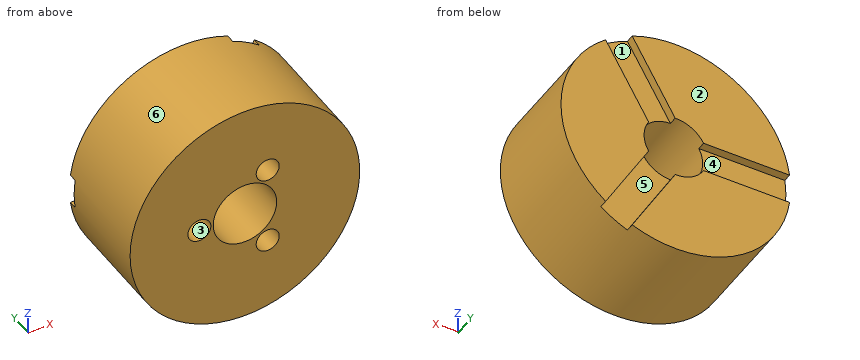
Autodesk Inventor part; units mm, degrees
ref_plane "XZ Plane" through (0, 0, 0) normal (0, 1, 0) x (-1, 0, 0)
sketch "Sketch1" plane through (0, 0, 0) normal (0, 1, 0) x (-1, 0, 0)
  circle A0 centre (0, 0) radius 99.7
extrude "Extrusion1" add sketch "Sketch1" along normal blind 90.9
sketch "Sketch2" plane through (0, 90.9, 0) normal (0, 1, 0) x (1, 0, 0)
  circle A0 centre (0, 0) radius 27.56
  dimension "d3" = 55.12
extrude "Extrusion2" cut sketch "Sketch2" against normal blind 90.9
sketch "Sketch3" plane through (0, 90.9, 0) normal (0, 1, 0) x (1, 0, 0)
  circle A0 centre (0, 0) radius 99.7
  line L0 (-99.7, 0) -> (-98.8062, 13.32)
  line L1 (-98.8062, 13.32) -> (-24.1274, 13.32)
  circle A1 centre (0, 0) radius 27.56
  line L2 (-99.7, 0) -> (-98.8062, -13.32)
  line L3 (-98.8062, -13.32) -> (-24.1274, -13.32)
  line L4 (37.8676, -92.2287) -> (0.5282, -27.5549)
  line L5 (49.85, -86.3427) -> (37.8676, -92.2287)
  line L6 (49.85, -86.3427) -> (60.9386, -78.9087)
  line L7 (60.9386, -78.9087) -> (23.5992, -14.2349)
  line L8 (60.9386, 78.9087) -> (23.5992, 14.2349)
  line L9 (49.85, 86.3427) -> (60.9386, 78.9087)
  line L10 (49.85, 86.3427) -> (37.8676, 92.2287)
  line L11 (37.8676, 92.2287) -> (0.5282, 27.5549)
  line L12 (-24.1274, 13.32) -> (-24.1274, -13.32)
  line L13 (0.5282, 27.5549) -> (23.5992, 14.2349)
  line L14 (23.5992, -14.2349) -> (0.5282, -27.5549)
  dimension "d6" = 13.35
  dimension "d15" = 360
ref_plane "Work Plane2" through (-99.7, 83.72, 0) normal (0.9978, 0, 0.067) x (0.067, 0, -0.9978)
sketch "Sketch4" plane through (-99.7, 83.72, 0) normal (0.9978, 0, 0.067) x (0.067, 0, -0.9978)
  line L0 (13.35, 0) -> (13.35, 7.18)
  line L1 (-13.2303, 7.18) -> (-13.2303, 0)
  point P0 (6.675, -83.72)
ref_plane "Work Plane1" through (-98.8062, 83.72, 13.32) normal (0.9978, 0, -0.067) x (-0.067, 0, -0.9978)
sketch "Sketch5" plane through (-98.8062, 83.72, 13.32) normal (0.9978, 0, -0.067) x (-0.067, 0, -0.9978)
  line L0 (13.35, 0) -> (13.35, 7.18)
  line L1 (0, 0) -> (13.35, 0)
  line L2 (13.35, 5.7337) -> (13.35, 0)
  line L3 (13.35, 0) -> (0, 0)
  line L4 (0, 0) -> (0, 7.18)
  line L5 (0, 7.18) -> (0, 0)
  line L6 (106.375, 7.18) -> (-93.025, 7.18)
  point P0 (6.675, -83.72)
  point P1 (26.5803, 7.18)
extrude "Extrusion4" cut sketch "Sketch5" against normal blind 7.18
ref_plane "Work Plane3" through (-99.7, 83.72, 0) normal (0.9978, 0, 0.067) x (0.067, 0, -0.9978)
sketch "Sketch6" plane through (-99.7, 83.72, 0) normal (0.9978, 0, 0.067) x (0.067, 0, -0.9978)
  line L0 (0, 0) -> (13.35, 0)
  line L1 (0, 0) -> (0, 7.18)
  line L2 (0, 0) -> (0, 7.18)
  line L3 (13.35, 7.18) -> (18.3498, 7.18)
  line L4 (0, 7.18) -> (13.35, 7.18)
  line L5 (13.35, 0) -> (13.35, 7.18)
  line L6 (13.35, 7.18) -> (13.35, 0)
  line L7 (13.35, 0) -> (0, 0)
  point P0 (6.675, -83.72)
extrude "Extrusion5" cut sketch "Sketch6" against normal blind 7.18
extrude "Extrusion6" cut sketch "Sketch3" against normal blind 7.18 contours L8 A1 L11 L10 L9 | L6 L5 L4 A1 L7 | L13 A1 | A1 L14 | L1 A1 L3 L2 L0
sketch "Sketch7" plane through (49.85, 83.72, -86.3427) normal (-0.5569, 0, 0.8306) x (0.8306, 0, 0.5569)
  line L0 (13.35, 7.18) -> (0, 7.18)
  line L1 (13.35, 0) -> (13.35, 7.18)
  line L2 (0, 7.18) -> (13.35, 7.18)
  line L3 (13.35, 0) -> (18.3498, 0)
  line L4 (13.35, 7.18) -> (13.35, 0)
  line L5 (0, 7.18) -> (0, 0)
  line L6 (13.35, 0) -> (0, 0)
  line L7 (0, 0) -> (0, 6.2119)
  line L8 (0, 7.18) -> (-13.2303, 7.18)
  line L9 (-13.2303, 4.6736) -> (0, 7.18)
  line L10 (0, 7.18) -> (0, 0)
  line L11 (-13.2303, -2.9965) -> (-13.2303, 4.6736)
  line L12 (-13.2303, 0) -> (-13.2303, 7.18)
  point P0 (6.675, -83.72)
extrude "Extrusion7" cut sketch "Sketch7" against normal blind 10 contours L1 L6 L5 L0
sketch "Sketch8" plane through (37.8676, 83.72, -92.2287) normal (-0.4409, 0, 0.8976) x (0.8976, 0, 0.4409)
  line L0 (0, 0) -> (0, 7.18)
  line L1 (-4.9998, 0) -> (0, 0)
  line L2 (0, 7.18) -> (0, 0)
  line L3 (0, 0) -> (13.35, 0)
  line L4 (0, 0) -> (13.35, 0)
  line L5 (13.35, 7.18) -> (13.35, 0)
  line L6 (13.35, 0) -> (13.35, 7.18)
  line L7 (0, 7.18) -> (13.35, 7.18)
  line L8 (13.35, 7.18) -> (0, 7.18)
  line L9 (0, 7.18) -> (0, 4.7035)
  point P0 (6.675, -83.72)
extrude "Extrusion8" cut sketch "Sketch8" against normal blind 10
sketch "Sketch10" plane through (49.85, 83.72, 86.3427) normal (-0.4409, 0, -0.8976) x (-0.8976, 0, 0.4409)
  line L0 (0, 7.18) -> (13.35, 7.18)
  line L1 (13.35, 7.18) -> (18.3498, 7.18)
  line L2 (0, 7.18) -> (13.35, 7.18)
  line L3 (13.35, 0) -> (18.3498, 0)
  line L4 (13.35, 7.18) -> (13.35, 0)
  line L5 (0, 0) -> (13.35, 0)
  line L6 (13.35, 0) -> (0, 0)
  line L7 (0, 0) -> (0, 7.18)
  line L8 (0, 7.18) -> (0, 0)
  point P0 (6.675, -83.72)
extrude "Extrusion9" cut sketch "Sketch10" against normal blind 10
sketch "Sketch11" plane through (60.9386, 83.72, 78.9087) normal (-0.5569, 0, -0.8306) x (-0.8306, 0, 0.5569)
  line L0 (-4.9998, 7.18) -> (0, 7.18)
  line L1 (13.35, 7.18) -> (0, 7.18)
  line L2 (0, 7.18) -> (13.35, 7.18)
  line L3 (0, 0) -> (13.35, 0)
  line L4 (13.35, 7.18) -> (13.35, 0)
  line L5 (13.35, 0) -> (0, 0)
  line L6 (0, 0) -> (0, 7.18)
  line L7 (0, 0) -> (0, 7.18)
  point P0 (6.675, -83.72)
extrude "Extrusion10" cut sketch "Sketch11" against normal blind 10
sketch "Sketch12" plane through (0, 90.9, 0) normal (0, 1, 0) x (1, 0, 0)
  arc A0 (37.8676, -92.2287) -> (60.9386, -78.9087) centre (0, 0) ccw
  arc A1 (-98.8062, -13.32) -> (37.8676, -92.2287) centre (0, 0) ccw
  arc A2 (-98.8062, 13.32) -> (-98.8062, -13.32) centre (0, 0) ccw
  arc A3 (37.8676, 92.2287) -> (-98.8062, 13.32) centre (0, 0) ccw
  arc A4 (60.9386, 78.9087) -> (37.8676, 92.2287) centre (0, 0) ccw
  arc A5 (60.9386, -78.9087) -> (60.9386, 78.9087) centre (0, 0) ccw
  circle A6 centre (0, 0) radius 99.7
ref_plane "Work Plane5" through (-99.7, 0, 0) normal (1, 0, 0) x (0, 1, 0)
ref_plane "Work Plane6" through (0, 0, -99.7) normal (0, 0, 1) x (1, 0, 0)
sketch "Sketch13" plane through (0, 83.72, 0) normal (0, 1, 0) x (1, 0, 0)
  arc A0 (60.9386, 78.9087) -> (37.8676, 92.2287) centre (0, 0) ccw
sketch "Sketch14" plane through (-99.7, 83.72, 0) normal (0.9978, 0, 0.067) x (0.067, 0, -0.9978)
  point P0 (6.675, -83.72)
sketch "Sketch15" plane through (0, 0, 0) normal (0, -1, 0) x (1, 0, 0)
  circle A0 centre (0, 0) radius 27.56
  circle A1 centre (19.78, 34.26) radius 10
  circle A2 centre (-39.56, 0) radius 10
  circle A3 centre (19.78, -34.26) radius 10
  point P0 (0.5282, 27.5549)
  point P1 (23.5992, 14.2349)
  dimension "d32" = 360
extrude "Extrusion11" cut sketch "Sketch15" against normal blind 40 contours A1 | A2 | A3
properties part number "3 jaww"
Model file for the job. Use its own axes, mm. Face numbers are marked on the shaded views. A direction names the side the tool comes from. Give positions to 0.01 mm unless a question says otherwise; leave off trailing zeros. Write each loop counter-clockwise with the first axis right and the second up, starting at its lowest first coordinate (ties: lowest second). Pieces come first, ordered by that corner, then holes. Notation, with made-up numbers: (4.25, 40) - (41.25, 40) arc R34 cw to (41.25, 73) - close; hole circle Ø11 at (15.5, 56.25). An arc over 180 degrees is marked (long way). Answer as CSV lines item,"result".
1. Band-saw the part on A-A (x = 19.78). Write the cut outline in (y, z).
Responses:
outline,"(0, -97.72) - (90.9, -97.72) - (90.9, -60.9) - (83.72, -60.9) - (83.72, -19.19) - (0, -19.19) - (0, -24.26) - (40, -24.26) - (40, -44.26) - (0, -44.26) - close; (0, 19.19) - (83.72, 19.19) - (83.72, 60.9) - (90.9, 60.9) - (90.9, 97.72) - (0, 97.72) - (0, 44.26) - (40, 44.26) - (40, 24.26) - (0, 24.26) - close"
2. Two-plate mould, pull along X, no slides. Class the marked faces 4, 5 and 6: +X half, -X half, draft (parallel to the pull), parting line (faces both ways), or undercut.
Responses:
face 4,"draft"
face 5,"undercut"
face 6,"parting line"
3. Drill centre lines: L1, parallel to Z at x = 19.78, y = 31; L2, parallel to Z at x = 18, y = 19; L3, parallel to X at y = 13, z = 41. Where is each one in solid material? Low to high. Write a range as [from, to].
Responses:
L1,"z = [-97.72, -44.26], [-24.26, -19.19], [19.19, 24.26], [44.26, 97.72]"
L2,"z = [-98.06, -44.1], [-24.42, -20.87], [20.87, 24.42], [44.1, 98.06]"
L3,"x = [-90.88, 12.39], [27.17, 90.88]"
4. Band-saw the part on B-B (y = 18). Write the cut outline in (x, z).
Responses:
outline,"circle Ø199.4 at (0, 0); hole circle Ø20 at (-39.56, 0); hole circle Ø55.12 at (0, 0); hole circle Ø20 at (19.78, -34.26); hole circle Ø20 at (19.78, 34.26)"
5. Band-saw the part on D-D (y = 48). Write the cut outline in (x, z), and give its area (3 significant figures).
Responses:
outline,"circle Ø199.4 at (0, 0); hole circle Ø55.12 at (0, 0)"
area,"28,800 mm2"
6. 3-axis set-ups, long thin cutter, end or side, ignore diameter. For the marked faces 1, 2 and 3: which of +Z, -Z, +X, -X, +Y, -Y reach the whole face in a straight line?
Responses:
face 1,"+Y"
face 2,"+Z, -Z, +X, -X, +Y"
face 3,"-Y"
7. Pin check, flat tips, straight feed: pin 1 (6 mm diameter, centred on x = 19, z = -30.5, fed in from -Y); pin 2 (23 mm diameter, centred on x = -39.56, z = 0, fed in from +Y); pin 3 (2 mm diameter, centred on x = -75.5, y = 87.5, fed in from +Z). Stop position of each tip, or through.
Responses:
pin 1,"stops at y = 40"
pin 2,"stops at y = 83.72"
pin 3,"stops at z = 66.26"
8. Band-saw the part on C-C (z = 57.5). Write the cut outline in (x, y), and give its area (3 significant figures).
Responses:
outline,"(-81.45, 0) - (81.45, 0) - (81.45, 90.9) - (48.58, 90.9) - (48.58, 83.72) - (17.82, 83.72) - (17.82, 90.9) - (-81.45, 90.9) - close"
area,"14,600 mm2"
